from build123d import *

# Parameters (mm, degrees)
SKETCH_3_R      = 2
EXTRUDE_1_DEPTH = 1


with BuildPart() as part:
    # Эскиз3 → Бобышка-Вытянуть1 (new body)
    with BuildSketch(Plane.XY):
        with BuildLine():
            Line((10, 0), (60, 0))
            add(Edge.make_bspline(
                [(60, 0), (73.743685419, 0), (72.922981248, -10), (60, -10)],
                knots=[0, 0, 0, 0, 1, 1, 1, 1], degree=3))
            Line((60, -10), (10, -10))
            add(Edge.make_bspline(
                [(10, 0), (-3.743685419, 0), (-2.922981248, -10), (10, -10)],
                knots=[0, 0, 0, 0, 1, 1, 1, 1], degree=3))
        make_face()
        with Locations((5, -5)):
            Circle(SKETCH_3_R, mode=Mode.SUBTRACT)
        with Locations((65, -5)):
            Circle(SKETCH_3_R, mode=Mode.SUBTRACT)
        with Locations((15, -5)):
            Circle(SKETCH_3_R, mode=Mode.SUBTRACT)
        with Locations((25, -5)):
            Circle(SKETCH_3_R, mode=Mode.SUBTRACT)
        with Locations((35, -5)):
            Circle(SKETCH_3_R, mode=Mode.SUBTRACT)
        with Locations((45, -5)):
            Circle(SKETCH_3_R, mode=Mode.SUBTRACT)
        with Locations((55, -5)):
            Circle(SKETCH_3_R, mode=Mode.SUBTRACT)
    extrude(amount=EXTRUDE_1_DEPTH)


solid = part.part
Source: CAD feature listing. Evaluate the final solid. Frame: model axes, mm. Give positions to 0.01 mm unless a question says otherwise; leave off trailing zeros. Order: outer loops, then holes, each group sorted by start corner. A loop starts at its lowest first (then second) coordinate and runs counter-clockwise, first axis right, second up. Notation, with made-up numbers: (72, 26) -> (93, 26) arc R21 ccw to (93, 54) -> close; hole circle Ø7 at (22.25, 1). An arc over 180 degrees is marked (long way). Write item = value, one per line.
Q1. Cut plane B-B, the plane z = 0.7. State how many separate pieces and enclosed holes the cut face has, and give its area (3 significant figures).
Data:
separate_pieces = 1
enclosed_holes = 7
area = 572 mm^2
Q2. Pin query (flat end, axial travel): pin 1 (4.5 mm diameter, centred on x = 65, y = -5, fed in from -Z). Return the tip coordinate at first contact, or that it passes through.
Data:
pin_1 = 0
Q3. Material intervals for line 1 (Y direction, x = 25, z = 0.35); line 2 (Y direction, x = 6.5, z = 0.8); line 3 (X direction, y = -1.25, z = 0.35), sorted ascending. Write a range as from..to.
Data:
line_1 = -10..-7, -3..0
line_2 = -9.72..-6.32, -3.68..-0.25
line_3 = 2.99..67.01
Q4. Pull-direction query (Y, two-part tool) for faces 1 (the face through (3.4, -6.2, 0.5)), 2 (the face through (36, -3, 0)); classes: released by +Y, released by -Y, zero draft, split by the parting line, or undercut.
Data:
face_1 = undercut
face_2 = zero draft
Q5. Cut plane A-A, the plane x = 25. Output: boundary loops of the cut face in (y, z), and give its area (3 significant figures).
Data:
outline = (-10, 0) -> (-7, 0) -> (-7, 1) -> (-10, 1) -> close; (-3, 0) -> (0, 0) -> (0, 1) -> (-3, 1) -> close
area = 6.00 mm^2
